Part model, mm, in its own coordinate system. Round coordinates to 2 decimals unless told otherwise and drop trailing zeros. Write each loop counter-clockwise with the first axis right and the second up, starting at its lowest first coordinate (ties: lowest second). Pieces come first, ordered by that corner, then holes. Notation, with made-up numbers: M -19,-20 L 0,-20 A24 cw 0,-3 Z; hole C 82,-11.5 d1. An arc over 180 degrees is marked long. Use one line per item in the form item = value. Start each with the question number.
Item 1: Flat gauge pins, fed straight in: pin 1 Ø1.5 at (y, z) = (-57, 3) entering from -X; pin 2 Ø3 at (x, z) = (-351.5, 2) entering from +Y; pin 3 Ø1.5 at (y, z) = (-54.5, 3) entering from +X. Where does each tip first touch, or does it go through?
Item 2: Probe L1, parallel to X at y = -56, z = 1.3. List the from-to ranges inside material, lowest first.
Item 3: Cut at A-A, the plane y = -43. Give the cut face in (x, z).
from build123d import *

# Parameters (mm, degrees)
SKETCH1_W           = 405
SKETCH1_H           = 100
BOSS_EXTRUDE1_DEPTH = 5
SKETCH2_W           = 5
SKETCH2_H           = 5
CUT_EXTRUDE1_DEPTH  = 5
BOSS_EXTRUDE2_DEPTH = 5
SKETCH6_W           = 15
SKETCH6_H           = 50
CUT_EXTRUDE4_DEPTH  = 5


with BuildPart() as part:
    # Sketch1 → Boss-Extrude1 (new body)
    with BuildSketch(Plane.XY):
        with Locations((-202.5, -50)):
            Rectangle(SKETCH1_W, SKETCH1_H)
    extrude(amount=BOSS_EXTRUDE1_DEPTH)

    # Sketch2 → Cut-Extrude1 (cut)
    with BuildSketch(Plane.XY.offset(5)):
        with Locations((-402.5, -77.5)):
            Rectangle(SKETCH2_W, SKETCH2_H)
        with Locations((-402.5, -22.5)):
            Rectangle(SKETCH2_W, SKETCH2_H)
        with Locations((-2.5, -22.5)):
            Rectangle(SKETCH2_W, SKETCH2_H)
        with Locations((-2.5, -77.5)):
            Rectangle(SKETCH2_W, SKETCH2_H)
    extrude(amount=-CUT_EXTRUDE1_DEPTH, mode=Mode.SUBTRACT)

    # Sketch3 → Boss-Extrude2 (add)
    with BuildSketch(Plane.XY.offset(5)):
        Polygon((-405, -30), (-405, -25), (-415, -25), (-415, -75), (-405, -75), (-405, -70), (-410, -70), (-410, -30), align=None)
        Polygon((0, -30), (5, -30), (5, -70), (0, -70), (0, -75), (10, -75), (10, -25), (0, -25), align=None)
    extrude(amount=-BOSS_EXTRUDE2_DEPTH)

    # Sketch6 → Cut-Extrude4 (cut)
    with BuildSketch(Plane.XY.offset(5)):
        with Locations((2.5, -50)):
            Rectangle(SKETCH6_W, SKETCH6_H)
        with Locations((-407.5, -50)):
            Rectangle(SKETCH6_W, SKETCH6_H)
    extrude(amount=-CUT_EXTRUDE4_DEPTH, mode=Mode.SUBTRACT)


solid = part.part
Model answer:
q1.pin_1 = -400
q1.pin_2 = 0
q1.pin_3 = -5
q2.L1 = -400 to -5
q3.outline = M -400,0 L -5,0 L -5,5 L -400,5 Z
